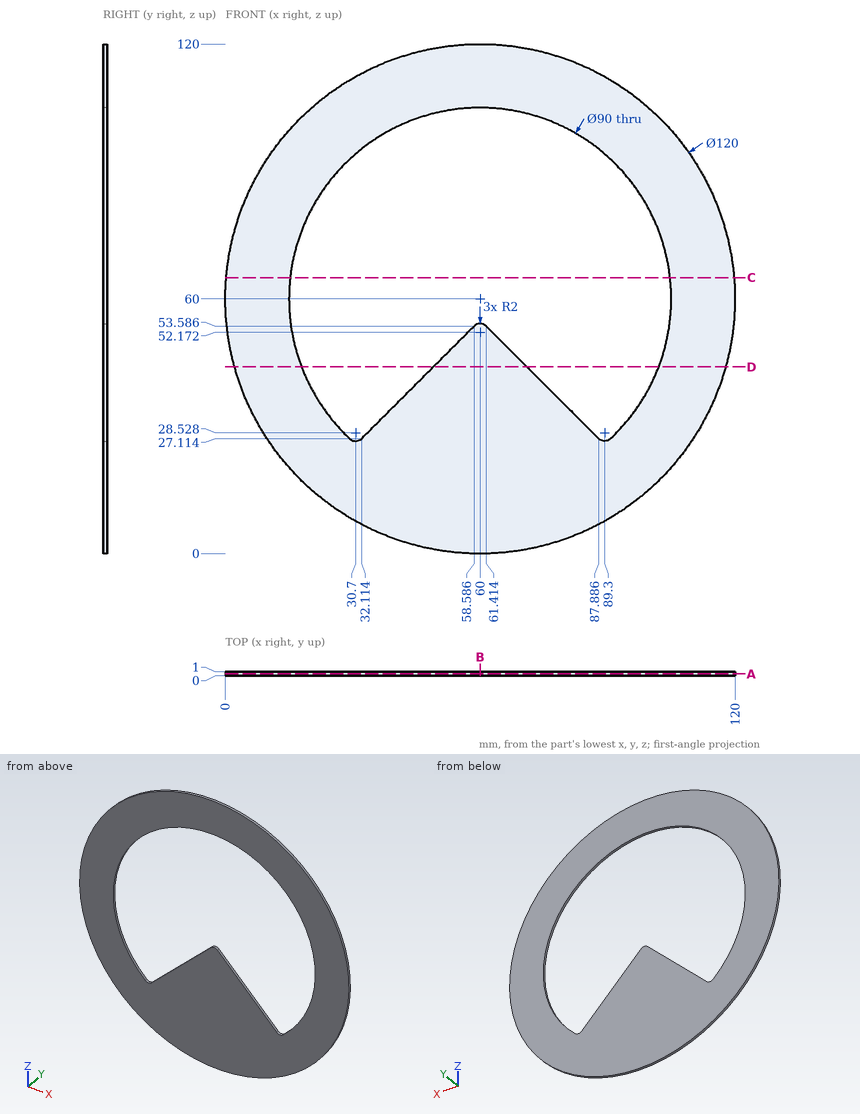
Job drawing, mm, ordinate dimensions from the low corner. One solid piece. Give positions to 0.01 mm unless a question says otherwise; leave off trailing zeros. Loops run counter-clockwise (first coordinate to the right, second up) from the corner with the lowest first, then second, coordinate; pieces in that order, holes last. Notation, with made-up numbers: (81, -13.75) -> (122, -13.75) arc R17 ccw to (122, -6.75) -> close; hole circle Ø9 at (27, 76). An arc over 180 degrees is marked (long way). Write each question's results on one line, items separated by ' | '.
(1) Cut at B-B on x = 60. List the corners of the cut face in (y, z).
Geometry results:
outline: (0, 0) -> (1, 0) -> (1, 54.17) -> (0, 54.17) -> close; (0, 105) -> (1, 105) -> (1, 120) -> (0, 120) -> close
(2) Flat gauge pin, fed straight in: pin 1 Ø10 at (x, z) = (96, 59.5) entering from +Y. Where does the tip first touch, or does it go through?
Geometry results:
pin 1: passes through
(3) Cut at A-A on y = 0.5. List the corners of the cut face in (x, z) (1 decimal).
Geometry results:
outline: circle Ø120 at (60, 60); hole (29.3, 27.1) arc R2 ccw to (32.1, 27.1) -> (58.6, 53.6) arc R2 cw to (61.4, 53.6) -> (87.9, 27.1) arc R2 ccw to (90.7, 27.1) arc R45 ccw (long way) to start
(4) Cut at D-D on z = 44. List the corners of the cut face in (x, y).
Geometry results:
outline: (2.17, 0) -> (17.94, 0) -> (17.94, 1) -> (2.17, 1) -> close; (49, 0) -> (71, 0) -> (71, 1) -> (49, 1) -> close; (102.06, 0) -> (117.83, 0) -> (117.83, 1) -> (102.06, 1) -> close
(5) Cut at C-C on z = 65. List the corners of the cut face in (x, y).
Geometry results:
outline: (0.21, 0) -> (15.28, 0) -> (15.28, 1) -> (0.21, 1) -> close; (104.72, 0) -> (119.79, 0) -> (119.79, 1) -> (104.72, 1) -> close
(6) Probe line 1 along X through (y, z) = (0.75, 43) (1 decimal); line 2 along X through (y, z) = (0.7, 59); line 3 along Z through (x, y) = (53.5, 0.65) (1 decimal). List the from-to ranges inside material, lowest first.
Geometry results:
line 1: x = 2.5 to 18.3, 48 to 72, 101.7 to 117.5 | line 2: x = 0.01 to 15.01, 104.99 to 119.99 | line 3: z = 0.4 to 48.5, 104.5 to 119.6
